from build123d import *

# Parameters (mm, degrees)
F0_W      = 27
F0_H      = 15.9
F0_W_2    = 15.9
F0_H_2    = 27
F0_W_3    = 3
F0_H_3    = 3
F1_DEPTH  = 21.9
F2_DEPTH  = 51.8
F3_R      = 7.95
F6_DEPTH  = 30
F7_DEPTH  = 30
F4_R      = 7.9
F8_DEPTH  = 30
F12_DEPTH = 58.2
F13_DEPTH = 58.2
F14_DEPTH = 30


with BuildPart() as f1:
    # F0 (on Front) → F1 (new body)
    with BuildSketch(Plane.XZ):
        with BuildLine():
            Line((-34.3576915575, 15.9), (-42.3076915575, 15.9))
            Line((-42.3076915575, 15.9), (-42.3076915575, 7.9499999931))
            ThreePointArc((-42.3076915575, 7.9499999931), (-39.9791904704, 13.571498908), (-34.3576915575, 15.9))
        make_face()
        with BuildLine():
            ThreePointArc((-34.3576915575, 15.9), (-39.9791904704, 13.571498908), (-42.3076915575, 7.9499999931))
            ThreePointArc((-42.3076915575, 7.9499999931), (-39.9791904655, 2.3285010871), (-34.3576915575, 0))
            ThreePointArc((-34.3576915575, 0), (-28.7361926471, 2.3285010896), (-26.4076915575, 7.95))
            ThreePointArc((-26.4076915575, 7.95), (-28.7361926471, 13.5714989104), (-34.3576915575, 15.9))
        make_face()
        Polygon((-42.3076915575, 18.9), (-42.3076915575, 45.9), (-26.4076915575, 45.9), (-26.4076915575, 18.9), (-23.4076915575, 18.9), (-23.4076915575, 48.9), (-45.3076915575, 48.9), (-45.3076915575, 18.9), align=None)
        with Locations((-9.9076915575, 7.95)):
            Rectangle(F0_W, F0_H)
        with Locations((-34.3576915575, 32.4)):
            Rectangle(F0_W_2, F0_H_2)
        with BuildLine():
            ThreePointArc((-34.3576915575, 0), (-39.9791904655, 2.3285010871), (-42.3076915575, 7.9499999931))
            Line((-42.3076915575, 7.9499999931), (-42.3076915575, 0))
            Line((-42.3076915575, 0), (-34.3576915575, 0))
        make_face()
        with BuildLine():
            Line((-26.4076915575, 0), (-26.4076915575, 7.95))
            ThreePointArc((-26.4076915575, 7.95), (-28.7361926471, 2.3285010896), (-34.3576915575, 0))
            Line((-34.3576915575, 0), (-26.4076915575, 0))
        make_face()
        with BuildLine():
            Line((-26.4076915575, 7.95), (-26.4076915575, 15.9))
            Line((-26.4076915575, 15.9), (-34.3576915575, 15.9))
            ThreePointArc((-34.3576915575, 15.9), (-28.7361926471, 13.5714989104), (-26.4076915575, 7.95))
        make_face()
        Polygon((6.5923084425, 18.9), (-23.4076915575, 18.9), (-23.4076915575, 15.9), (3.5923084425, 15.9), (3.5923084425, 0), (-23.4076915575, 0), (-23.4076915575, -3), (6.5923084425, -3), align=None)
        Polygon((-26.4076915575, 18.9), (-42.3076915575, 18.9), (-42.3076915575, 15.9), (-34.3576915575, 15.9), (-26.4076915575, 15.9), align=None)
        Polygon((-23.4076915575, 15.9), (-26.4076915575, 15.9), (-26.4076915575, 7.95), (-26.4076915575, 0), (-23.4076915575, 0), align=None)
        Polygon((-42.3076915575, 15.9), (-42.3076915575, 18.9), (-45.3076915575, 18.9), (-45.3076915575, -3), (-23.4076915575, -3), (-23.4076915575, 0), (-26.4076915575, 0), (-34.3576915575, 0), (-42.3076915575, 0), (-42.3076915575, 7.9499999931), align=None)
        with Locations((-24.9076915575, 17.4)):
            Rectangle(F0_W_3, F0_H_3)
    extrude(amount=F1_DEPTH)

    # F0 (on Front) → F2 (join)
    with BuildSketch(Plane.XZ):
        Polygon((-42.3076915575, 15.9), (-42.3076915575, 18.9), (-45.3076915575, 18.9), (-45.3076915575, -3), (-23.4076915575, -3), (-23.4076915575, 0), (-26.4076915575, 0), (-34.3576915575, 0), (-42.3076915575, 0), (-42.3076915575, 7.9499999931), align=None)
        with BuildLine():
            ThreePointArc((-34.3576915575, 15.9), (-39.9791904704, 13.571498908), (-42.3076915575, 7.9499999931))
            ThreePointArc((-42.3076915575, 7.9499999931), (-39.9791904655, 2.3285010871), (-34.3576915575, 0))
            ThreePointArc((-34.3576915575, 0), (-28.7361926471, 2.3285010896), (-26.4076915575, 7.95))
            ThreePointArc((-26.4076915575, 7.95), (-28.7361926471, 13.5714989104), (-34.3576915575, 15.9))
        make_face()
        Polygon((-26.4076915575, 18.9), (-42.3076915575, 18.9), (-42.3076915575, 15.9), (-34.3576915575, 15.9), (-26.4076915575, 15.9), align=None)
        Polygon((-23.4076915575, 15.9), (-26.4076915575, 15.9), (-26.4076915575, 7.95), (-26.4076915575, 0), (-23.4076915575, 0), align=None)
        with Locations((-24.9076915575, 17.4)):
            Rectangle(F0_W_3, F0_H_3)
        with BuildLine():
            Line((-26.4076915575, 7.95), (-26.4076915575, 15.9))
            Line((-26.4076915575, 15.9), (-34.3576915575, 15.9))
            ThreePointArc((-34.3576915575, 15.9), (-28.7361926471, 13.5714989104), (-26.4076915575, 7.95))
        make_face()
        with BuildLine():
            Line((-34.3576915575, 15.9), (-42.3076915575, 15.9))
            Line((-42.3076915575, 15.9), (-42.3076915575, 7.9499999931))
            ThreePointArc((-42.3076915575, 7.9499999931), (-39.9791904704, 13.571498908), (-34.3576915575, 15.9))
        make_face()
        with BuildLine():
            ThreePointArc((-34.3576915575, 0), (-39.9791904655, 2.3285010871), (-42.3076915575, 7.9499999931))
            Line((-42.3076915575, 7.9499999931), (-42.3076915575, 0))
            Line((-42.3076915575, 0), (-34.3576915575, 0))
        make_face()
        with BuildLine():
            Line((-26.4076915575, 0), (-26.4076915575, 7.95))
            ThreePointArc((-26.4076915575, 7.95), (-28.7361926471, 2.3285010896), (-34.3576915575, 0))
            Line((-34.3576915575, 0), (-26.4076915575, 0))
        make_face()
    extrude(amount=F2_DEPTH)

    # F3 (on face) → F6 (cut)
    with BuildSketch(Plane.XZ.offset(51.8)):
        with Locations((-34.3576915575, 7.95)):
            Circle(F3_R)
    extrude(amount=-F6_DEPTH, mode=Mode.SUBTRACT)

    # F5 (on face) → F7 (cut)
    with BuildSketch(Plane.YZ.offset(6.5923084425)):
        with BuildLine():
            ThreePointArc((-3, 7.95), (-5.3285010896, 13.5714989104), (-10.95, 15.9))
            ThreePointArc((-10.95, 15.9), (-16.5714989104, 13.5714989104), (-18.9, 7.95))
            ThreePointArc((-18.9, 7.95), (-16.5714989104, 2.3285010896), (-10.95, 0))
            ThreePointArc((-10.95, 0), (-5.3285010896, 2.3285010896), (-3, 7.95))
        make_face()
    extrude(amount=-F7_DEPTH, mode=Mode.SUBTRACT)

    # F4 (on face) → F8 (cut)
    with BuildSketch(Plane.XY.offset(48.9)):
        with Locations((-34.3576915575, -10.9)):
            Circle(F4_R)
    extrude(amount=-F8_DEPTH, mode=Mode.SUBTRACT)

    # F10 (on face) → F12 (join)
    with BuildSketch(Plane.XZ.offset(51.8)):
        Polygon((-45.3076915575, -9.3), (-45.3076915575, -6.3), (-48.6076915575, -6.3), (-48.6076915575, 7), (-51.6076915575, 7), (-51.6076915575, -9.3), align=None)
        Polygon((-42.255833745, -3), (-45.3076915575, -3), (-45.3076915575, -6.3), (-45.3076915575, -9.3), (-29.0076915575, -9.3), (-29.0076915575, -6.3), (-42.255833745, -6.3), align=None)
    extrude(amount=-F12_DEPTH)

    # F11 (on face) → F13 (join, through all)
    with BuildSketch(Plane.YZ.offset(6.5923084425)):
        Polygon((0, -6.3), (0, -3), (-3, -3), (-3, -6.3), (-16.3, -6.3), (-16.3, -9.3), (0, -9.3), align=None)
        Polygon((3.3, -6.3), (0, -6.3), (0, -9.3), (6.3, -9.3), (6.3, 7), (3.3, 7), align=None)
    extrude(amount=-F13_DEPTH)

    # F10 (on face) → F14 (cut)
    with BuildSketch(Plane.XZ.offset(51.8)):
        Polygon((-45.3076915575, -9.3), (-45.3076915575, -6.3), (-48.6076915575, -6.3), (-48.6076915575, 7), (-51.6076915575, 7), (-51.6076915575, -9.3), align=None)
    extrude(amount=-F14_DEPTH, mode=Mode.SUBTRACT)


solid = f1.part
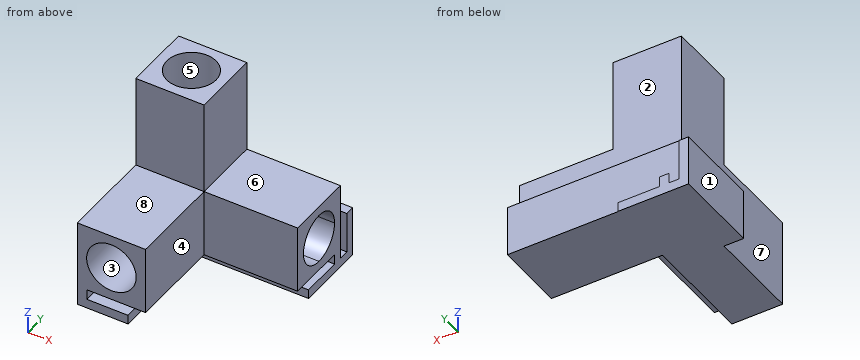
Design review of the part built by this model. Coordinates are the model's own, in mm. Face numbers are marked on the shaded views. A direction names the side the tool comes from. Round coordinates to 2 decimals unless told otherwise and drop trailing zeros. Write each loop counter-clockwise with the first axis right and the second up, starting at its lowest first coordinate (ties: lowest second). Pieces come first, ordered by that corner, then holes.
Item 1: Draft analysis for pull direction X (two halves, no side actions). For the marked faces 1, 2 and 3, state which applies: released by +X, released by -X, zero draft, split by the parting line, or undercut.
Item 2: Consider section B-B on z = -2. Give the boundary of the cut face in (x, y).
Item 3: Consider section C-C on y = -33. Give the boundary of the cut face in (x, z), and give its area (3 significant figures).
Item 4: For the marked faces 4, 5, 6, 7 and 8, list the 3-axis set-ups (+Z, -Z, +X, -X, +Y, -Y) from which the entire face can be reached by the end or side of a thin tool; tool diameter is ignored.
Item 5: Wall thickness on L1, parallel to Y at x = -4.5, z = 5; L2, parallel to Z at x = 1.5, y = -4; L3, parallel to Y at x = -18, z = -1: over which ranges is each line inside the solid? List them lowest first.
Item 6: For pin 1 Ø6.5 at (x, y) = (-7.5, -7) entering from +Z; pin 2 Ø8 at (y, z) = (-14, 11.5) entering from -X; pin 3 Ø11 at (y, z) = (-15.5, 27.5) entering from +X, all flat-tipped, find the tip position at first contact; note any pin that passes through.
Item 7: Consider section A-A on x = -15. Give the boundary of the cut face in (y, z).
Item 8: Consider section D-D on z = 29. Give the boundary of the cut face in (x, y).
Check values:
1. face 1: released by -X
1. face 2: zero draft
1. face 3: undercut
2. outline: (-51.61, -21.8) - (-48.61, -21.8) - (-48.61, 3.3) - (6.59, 3.3) - (6.59, 6.3) - (-48.61, 6.3) - (-48.61, 6.4) - (-51.61, 6.4) - close; (-45.31, -51.8) - (-23.41, -51.8) - (-23.41, -21.9) - (6.59, -21.9) - (6.59, 0) - (-45.31, 0) - close
3. outline: (-45.31, -9.3) - (-29.01, -9.3) - (-29.01, -6.3) - (-42.26, -6.3) - (-42.26, -3) - (-23.41, -3) - (-23.41, 18.9) - (-45.31, 18.9) - close; hole circle Ø15.9 at (-34.36, 7.95)
3. area: 340 mm2
4. face 4: +Z, -Z, +X, -Y
4. face 5: +Z
4. face 6: +Z, +X, +Y, -Y
4. face 7: +Z, -Y
4. face 8: +Z, +X, -X, -Y
5. L1: y = -21.9 to -18.33, -3.57 to 0, 3.3 to 6.3
5. L2: z = -9.3 to -6.3, -3 to 4.09, 11.81 to 18.9
5. L3: y = -21.9 to 0, 3.3 to 6.3
6. pin 1: stops at z = 18.9
6. pin 2: stops at x = -45.31
6. pin 3: stops at x = -23.41
7. outline: (-21.9, -3) - (-3, -3) - (-3, -6.3) - (-16.3, -6.3) - (-16.3, -9.3) - (6.3, -9.3) - (6.3, 7) - (3.3, 7) - (3.3, -6.3) - (0, -6.3) - (0, 18.9) - (-21.9, 18.9) - close; hole circle Ø15.9 at (-10.95, 7.95)
8. outline: (-45.31, -21.9) - (-23.41, -21.9) - (-23.41, 0) - (-45.31, 0) - close; hole circle Ø15.8 at (-34.36, -10.9)
